Could you check a few things on this model? Use its own coordinates, in mm. Face numbers are marked on the shaded views. Coordinates: 2 decimals unless noted, no trailing zeros. Order: outer loops, then holes, each group sorted by start corner. A loop starts at its lowest first (then second) coordinate and runs counter-clockwise, first axis right, second up. Notation, with made-up numbers: (64.25, 84.25) - (88.25, 84.25) arc R28 ccw to (88.25, 116.25) - close; hole circle Ø3 at (-9, 61.5). An arc over 180 degrees is marked (long way). Answer as CSV lines item,"result". Start each with the question number.
1. Thinking about a two-plate mould opening in Z: for the marked faces 1 and 2, which applies, released by +Z, released by -Z, zero draft, split by the parting line, or undercut?
2. I want a section at A-A, the plane x = -21. List the corners of the cut face in (y, z) for me.
3. I want a section at C-C, the plane x = 21.5. List the corners of the cut face in (y, z) for me, and give its area (3 significant figures).
4. I want a section at B-B, the plane z = 6. List the corners of the cut face in (x, y) for me, and give its area (3 significant figures).
5. I need wall thicknesses on probe 1 along X at (y, z) = (3.3, 13.5); probe 2 along X at (y, z) = (2.2, 18); probe 3 along Y at (x, z) = (26, 30). Which ranges of each line are inside material? Lowest first, please.
6. For pin 1 (4.5 mm diameter, centred on x = -44, z = -10, fed in from -Y); pin 2 (4 mm diameter, centred on x = 20, z = 27, fed in from +Y); pin 3 (1.5 mm diameter, centred on x = -6, z = 34.5, fed in from +Y), each with a flat end and sliding along its axis, tell me the tip position at first contact or that it passes through.
from build123d import *

# Parameters (mm, degrees)
EXTRUDE_1_DEPTH     = 1.5
SKETCH_2_R          = 5
CUT_EXTRUDE_1_DEPTH = 0.5
SKETCH_11_R         = 2
SKETCH_11_W         = 12.230000073
SKETCH_11_H         = 11.974599949
EXTRUDE_5_DEPTH     = 2.539974634
SKETCH_13_R         = 2
SKETCH_13_W         = 4
SKETCH_13_H         = 10
TYPEC_2_DEPTH       = 5.7999746
LED_3_START         = -4.25
LED_3_DEPTH         = 2.75
LED_1_R             = 0.5
CUT_EXTRUDE_2_REACH = 75.743
SKETCH_15_R         = 2
EXTRUDE_START       = -4
SKETCH_16_R         = 4
SKETCH_16_R_2       = 1
EXTRUDE_4_DEPTH     = 2.5
LED_2_START         = -1.5
SKETCH_17_W         = 1
SKETCH_17_H         = 6
LED_2_DEPTH         = 0.5
SKETCH_18_W         = 40
SKETCH_18_H         = 3
EXTRUDE_2_DEPTH     = 3.5


with BuildPart() as part:
    # 草图1 → 凸台-拉伸1 (new body)
    with BuildSketch(Plane(origin=(0, 0, 0), x_dir=(1, 0, 0), z_dir=(0, 1, 0))):
        Polygon((-51.714401712, -9.454370264), (-55.816720774, -9.454370264), (-55.816720774, -21.428970213), (-51.714401712, -21.428970213), (-51.714401712, -47.841670238), (46.085598288, -47.841670238), (46.085598288, 16.958329762), (-51.714401712, 16.958329762), align=None)
    extrude(amount=EXTRUDE_1_DEPTH)

    # 草图2 → 防滑切除-拉伸1 (cut)
    with BuildSketch(Plane.XZ):
        with Locations(Location((-43.814401712, -9.058329762, 0), (0, 0, 270))):
            Circle(SKETCH_2_R)
        with Locations(Location((-43.814401712, 39.941670238, 0), (0, 0, 270))):
            Circle(SKETCH_2_R)
        with Locations(Location((38.185598288, 39.941670238, 0), (0, 0, 90))):
            Circle(SKETCH_2_R)
        with Locations(Location((38.185598288, -9.058329762, 0), (0, 0, 90))):
            Circle(SKETCH_2_R)
    extrude(amount=-CUT_EXTRUDE_1_DEPTH, mode=Mode.SUBTRACT)

    # 草图11 → 充电板档板凸台-拉伸5 (add)
    with BuildSketch(Plane.XZ):
        with Locations((-28.914401712, 29.928970213)):
            Circle(SKETCH_11_R)
        with Locations((-28.914401712, 0.954370264)):
            Circle(SKETCH_11_R)
        with Locations((-49.701720738, 15.441670239)):
            Rectangle(SKETCH_11_W, SKETCH_11_H)
    extrude(amount=-EXTRUDE_5_DEPTH)

    # 草图13 → TypeC支撑凸台-拉伸2 (add)
    with BuildSketch(Plane.XZ):
        with Locations(Location((-28.914401712, 29.928970213, 0), (0, 0, 90))):
            Circle(SKETCH_13_R)
        with Locations(Location((-28.914401712, 0.954370264, 0), (0, 0, 90))):
            Circle(SKETCH_13_R)
        with Locations((-46.466720701, 15.441670238)):
            Rectangle(SKETCH_13_W, SKETCH_13_H)
    extrude(amount=-TYPEC_2_DEPTH)

    # 草图14 → LED限位凸台-拉伸3 (add)
    with BuildSketch(Plane.XZ.offset(LED_3_START)):
        Polygon((45.085598288, 12.441670238), (45.085598288, 18.441670238), (46.085598288, 18.441670238), (46.085598288, 21.441670238), (42.085598288, 21.441670238), (42.085598288, 9.441670238), (46.085598288, 9.441670238), (46.085598288, 12.441670238), align=None)
    extrude(amount=LED_3_DEPTH)

    # LED限位圆角1
    led_1_edges = [part.edges().sort_by_distance(p)[0] for p in [
        (45.585598288, 4.25, 18.441670238),
        (45.585598288, 4.25, 12.441670238),
        (45.085598288, 4.25, 15.441670238),
        (-48.466720701, 5.7999746, 15.441670238),
    ]]
    fillet(led_1_edges, radius=LED_1_R)

    # 草图15 → 螺丝孔位切除-拉伸2 (cut, up to next)
    with BuildSketch(Plane.XZ, mode=Mode.PRIVATE) as cut_extrude_2_sk1:
        with Locations(Location((-43.814401712, -9.058329762, 0), (0, 0, 270))):
            Circle(SKETCH_15_R)
    cut_extrude_2_tool1 = extrude(cut_extrude_2_sk1.sketch, amount=-CUT_EXTRUDE_2_REACH, mode=Mode.PRIVATE) & part.part
    # 草图15 → 螺丝孔位切除-拉伸2 (cut, up to next)
    with BuildSketch(Plane.XZ, mode=Mode.PRIVATE) as cut_extrude_2_sk2:
        with Locations(Location((-43.814401712, 39.941670238, 0), (0, 0, 270))):
            Circle(SKETCH_15_R)
    cut_extrude_2_tool2 = extrude(cut_extrude_2_sk2.sketch, amount=-CUT_EXTRUDE_2_REACH, mode=Mode.PRIVATE) & part.part
    # 草图15 → 螺丝孔位切除-拉伸2 (cut, up to next)
    with BuildSketch(Plane.XZ, mode=Mode.PRIVATE) as cut_extrude_2_sk3:
        with Locations(Location((38.185598288, -9.058329762, 0), (0, 0, 270))):
            Circle(SKETCH_15_R)
    cut_extrude_2_tool3 = extrude(cut_extrude_2_sk3.sketch, amount=-CUT_EXTRUDE_2_REACH, mode=Mode.PRIVATE) & part.part
    # 草图15 → 螺丝孔位切除-拉伸2 (cut, up to next)
    with BuildSketch(Plane.XZ, mode=Mode.PRIVATE) as cut_extrude_2_sk4:
        with Locations(Location((38.185598288, 39.941670238, 0), (0, 0, 270))):
            Circle(SKETCH_15_R)
    cut_extrude_2_tool4 = extrude(cut_extrude_2_sk4.sketch, amount=-CUT_EXTRUDE_2_REACH, mode=Mode.PRIVATE) & part.part
    add(cut_extrude_2_tool1.solids().sort_by_distance((-43.814402, 0, -9.05833))[0], mode=Mode.SUBTRACT)
    add(cut_extrude_2_tool2.solids().sort_by_distance((-43.814402, 0, 39.94167))[0], mode=Mode.SUBTRACT)
    add(cut_extrude_2_tool3.solids().sort_by_distance((38.185598, 0, -9.05833))[0], mode=Mode.SUBTRACT)
    add(cut_extrude_2_tool4.solids().sort_by_distance((38.185598, 0, 39.94167))[0], mode=Mode.SUBTRACT)

    # 草图16 → 螺丝孔凸台-拉伸4 (add)
    # profile 1 of 4: a face of its own
    with BuildSketch(Plane.XZ.offset(EXTRUDE_START)):
        with Locations((38.185598288, -9.058329762)):
            Circle(SKETCH_16_R)
        with Locations((38.185598288, -9.058329762)):
            Circle(SKETCH_16_R_2, mode=Mode.SUBTRACT)
    # profile 2 of 4: a face of its own
    with BuildSketch(Plane.XZ.offset(EXTRUDE_START)):
        with Locations((38.185598288, 39.941670238)):
            Circle(SKETCH_16_R)
        with Locations((38.185598288, 39.941670238)):
            Circle(SKETCH_16_R_2, mode=Mode.SUBTRACT)
    # profile 3 of 4: a face of its own
    with BuildSketch(Plane.XZ.offset(EXTRUDE_START)):
        with Locations((-43.814401712, -9.058329762)):
            Circle(SKETCH_16_R)
        with Locations((-43.814401712, -9.058329762)):
            Circle(SKETCH_16_R_2, mode=Mode.SUBTRACT)
    # profile 4 of 4: a face of its own
    with BuildSketch(Plane.XZ.offset(EXTRUDE_START)):
        with Locations((-43.814401712, 39.941670238)):
            Circle(SKETCH_16_R)
        with Locations((-43.814401712, 39.941670238)):
            Circle(SKETCH_16_R_2, mode=Mode.SUBTRACT)
    extrude(amount=EXTRUDE_4_DEPTH)

    # 草图17 → LED灯嵌入切除-拉伸2 (cut)
    with BuildSketch(Plane.XZ.offset(LED_2_START)):
        with Locations((45.585598288, 15.441670238)):
            Rectangle(SKETCH_17_W, SKETCH_17_H)
    extrude(amount=LED_2_DEPTH, mode=Mode.SUBTRACT)

    # 草图18 → 散热板支撑凸台-拉伸2 (add)
    with BuildSketch(Plane(origin=(0, 1.5, 0), x_dir=(1, 0, 0), z_dir=(0, 1, 0))):
        with Locations((-5.814401712, 3.058329762)):
            Rectangle(SKETCH_18_W, SKETCH_18_H)
        with Locations((-5.814401712, -33.941670238)):
            Rectangle(SKETCH_18_W, SKETCH_18_H)
    extrude(amount=EXTRUDE_2_DEPTH)


solid = part.part
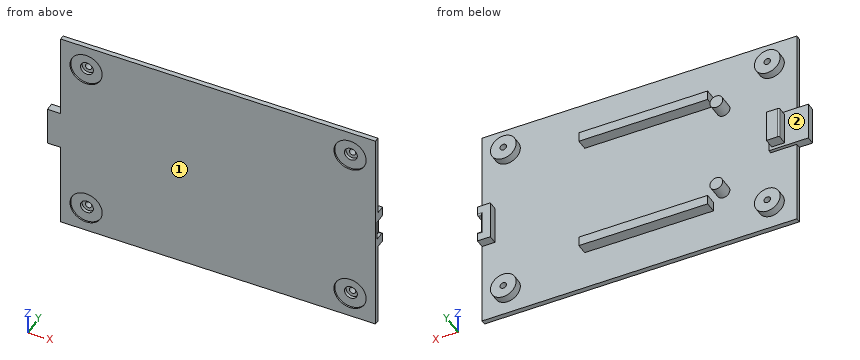
Solved:
1,face 1,"zero draft"
1,face 2,"undercut"
2,outline,"(0, -16.96) - (1.5, -16.96) - (1.5, -4.56) - (5, -4.56) - (5, -1.56) - (1.5, -1.56) - (1.5, 32.44) - (5, 32.44) - (5, 35.44) - (1.5, 35.44) - (1.5, 47.84) - (0, 47.84) - close"
3,outline,"(0, -16.96) - (1.5, -16.96) - (1.5, 47.84) - (0, 47.84) - close"
3,area,"97.2 mm2"
4,outline,"(-51.71, 0) - (46.09, 0) - (46.09, 1.5) - (-51.71, 1.5) - close"
4,area,"147 mm2"
5,probe 1,"x = -48.47 to -44.47, 42.09 to 45.09"
5,probe 2,"x = -55.82 to -43.59, 42.09 to 45.09"
5,probe 3,"y = 0 to 1.5"
6,pin 1,"stops at y = 0.5"
6,pin 2,"stops at y = 1.5"
6,pin 3,"stops at y = 5"
